```python
from build123d import *

# Parameters (mm, degrees)
BOSS_EXTRUDE1_DEPTH = 30
SKETCH3_OUTSIDE_W   = 54.806
SKETCH3_OUTSIDE_H   = 54.806
SKETCH3_OUTSIDE_W_2 = 20
SKETCH3_OUTSIDE_H_2 = 40
CUT_EXTRUDE1_DEPTH  = 20
CUT_EXTRUDE2_DEPTH  = 20


with BuildPart() as part:
    # Sketch2 → Boss-Extrude1 (new body)
    with BuildSketch(Plane(origin=(0, 0, 0), x_dir=(1, 0, 0), z_dir=(0, 1, 0))):
        with BuildLine():
            Line((-43.760683761, 14.358974359), (-43.760683761, -25.641025641))
            Line((-43.760683761, -25.641025641), (-13.760683761, -25.641025641))
            ThreePointArc((-13.760683761, -25.641025641), (-6.689615949, -22.712093453), (-3.760683761, -15.641025641))
            Line((-3.760683761, -15.641025641), (-3.760683761, -5.641025641))
            Line((-3.760683761, -5.641025641), (-13.760683761, -5.641025641))
            Line((-13.760683761, -5.641025641), (-13.760683761, 14.358974359))
            Line((-13.760683761, 14.358974359), (-43.760683761, 14.358974359))
        make_face()
    extrude(amount=BOSS_EXTRUDE1_DEPTH)

    # Sketch3 outside → Cut-Extrude1 (cut)
    with BuildSketch(Plane(origin=(0, 30, 0), x_dir=(1, 0, 0), z_dir=(0, 1, 0))):
        with Locations((-23.761, -5.641)):
            Rectangle(SKETCH3_OUTSIDE_W, SKETCH3_OUTSIDE_H)
        with Locations((-33.760683761, -5.641025641)):
            Rectangle(SKETCH3_OUTSIDE_W_2, SKETCH3_OUTSIDE_H_2, mode=Mode.SUBTRACT)
    extrude(amount=-CUT_EXTRUDE1_DEPTH, mode=Mode.SUBTRACT)

    # Sketch4 → Cut-Extrude2 (cut)
    with BuildSketch(Plane.ZY.offset(43.760683761)):
        Polygon((15.641025641, 30), (25.641025641, 20), (25.641025641, 30), align=None)
    extrude(amount=-CUT_EXTRUDE2_DEPTH, mode=Mode.SUBTRACT)


solid = part.part
```
Verification items for the finished model (mm, model axes). A direction names the side the tool comes from. Give positions to 0.01 mm unless a question says otherwise; leave off trailing zeros. Write each loop counter-clockwise with the first axis right and the second up, starting at its lowest first coordinate (ties: lowest second). Pieces come first, ordered by that corner, then holes. Notation, with made-up numbers: (23.25, 66) - (74.25, 66) arc R17 ccw to (74.25, 99) - close; hole circle Ø3 at (65, 62.5). An arc over 180 degrees is marked (long way). Put each result on its own line as item: value.
Q1. Section check D-D on z = 15. Record the cut outline in (x, y), and give its area (3 significant figures).
Result:
outline: (-43.76, 0) - (-3.76, 0) - (-3.76, 10) - (-23.76, 10) - (-23.76, 30) - (-43.76, 30) - close
area: 800 mm2
Q2. Section check C-C on y = 6.25. Record the cut outline in (x, z).
Result:
outline: (-43.76, -14.36) - (-13.76, -14.36) - (-13.76, 5.64) - (-3.76, 5.64) - (-3.76, 15.64) arc R10 ccw to (-13.76, 25.64) - (-43.76, 25.64) - close
Q3. Section check B-B on x = -30. Record the cut outline in (y, z), and give its area (3 significant figures).
Result:
outline: (0, -14.36) - (30, -14.36) - (30, 15.64) - (20, 25.64) - (0, 25.64) - close
area: 1,150 mm2
Q4. Section check A-A on z = -7. Record the cut outline in (x, y).
Result:
outline: (-43.76, 0) - (-13.76, 0) - (-13.76, 10) - (-23.76, 10) - (-23.76, 30) - (-43.76, 30) - close
Q5. Scan lines: probe 1 along X at (y, z) = (1, 5); probe 2 along X at (y, z) = (10.25, 19.5); probe 3 along Y at (x, z) = (-8, 7). Record each from-to range of solid material in increasing order. Write a range as from..to.
Result:
probe 1: -43.76..-13.76
probe 2: -43.76..-23.76
probe 3: 0..10
Q6. Set-up check for faces 1 (the face through (-13.761, 5, -4)), 2 (the face through (-23.761, 20, 6)), 3 (the face through (-34, 30, 0)): record each of +Z, -Z, +X, -X, +Y, -Y from which the full face is reachable in a straight line by a thin tool's end or side.
Result:
face 1: -Z, +X, +Y, -Y
face 2: +Z, -Z, +X, +Y
face 3: +Z, -Z, +X, -X, +Y
Q7. Depth check by flat-ended pin: P1, Ø12, axis at y = 14.5, z = 19, coming from the +X side; P2, Ø8, axis at x = -12.5, z = 1.5, coming from the +Y side; P3, Ø3, axis at x = -7.5, y = 7, coming from the -Z side; P4, Ø3, axis at y = 13.5, z = -10, coming from the +X side. Enter the tip coordinate at first touch or a pass-through.
Result:
P1: x = -3.76
P2: y = 10
P3: z = 5.64
P4: x = -23.76
